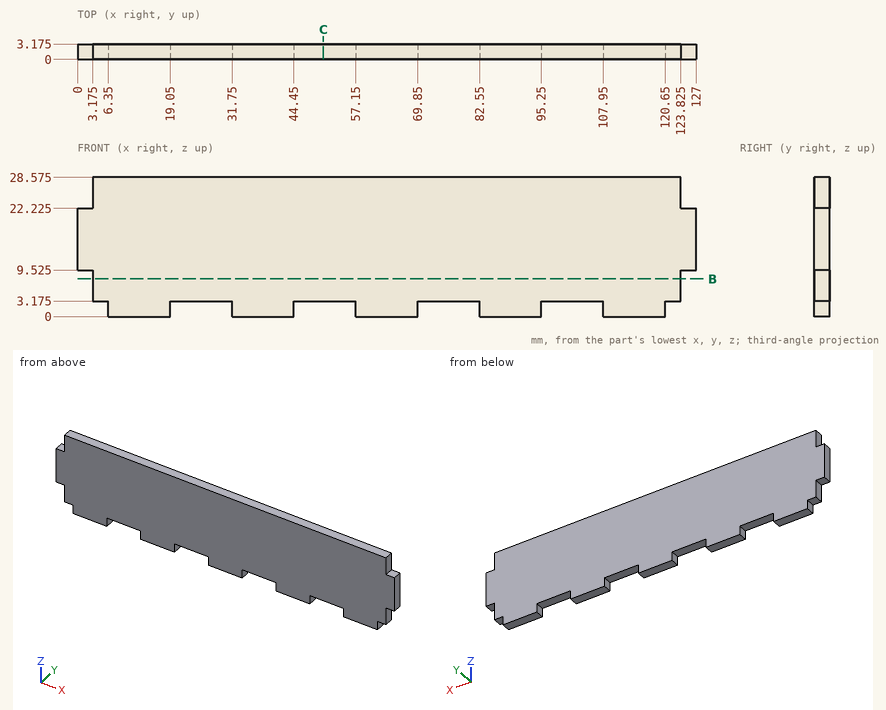
Could you check a few things on this drawing? It's one solid part, dimensions in mm from its lowest x, y, z. Give positions to 0.01 mm unless a question says otherwise; leave off trailing zeros. Loops run counter-clockwise (first coordinate to the right, second up) from the corner with the lowest first, then second, coordinate; pieces in that order, holes last. Notation, with made-up numbers: M -8.75,21 L -4.75,21 A23 cw -4.75,43 Z; hole C 10,-12 d9. An arc over 180 degrees is marked long. Answer as a JSON object with one key per item and string values.
Q1. Suppose I cut it at C-C, the plane x = 50.5. List the corners of the cut face in (y, z) for me (3 decimals).
Values found:
{"outline": "M 0,3.175 L 3.175,3.175 L 3.175,28.575 L 0,28.575 Z"}
Q2. Suppose I cut it at B-B, the plane z = 7.75. List the corners of the cut face in (x, y) for me (3 decimals).
Values found:
{"outline": "M 3.175,0 L 123.825,0 L 123.825,3.175 L 3.175,3.175 Z"}
Q3. For P1, Ø1, axis at x = 78, y = 0.5, coming from the -Z side (3 decimals); P2, Ø1.5, axis at y = 1.5, z = 3.5, coming from the -X side (3 decimals); P3, Ø1, axis at x = 2, y = 1.5, coming from the -Z side (3 decimals), each with a flat end and sliding along its axis, tell me the tip position at first contact or that it passes through.
Values found:
{"P1": "stops at z = 3.175", "P2": "stops at x = 3.175", "P3": "stops at z = 9.525"}
Q4. If I drill on probe 1 along X at (y, z) = (1.1, 3); probe 2 along Z at (x, y) = (28, 2.5) (3 decimals); probe 3 along X at (y, z) = (2, 8.75) (3 decimals), over which ranges is the centre line in solid material (lowest first)? Write a range as [from, to].
Values found:
{"probe 1": "x = [6.35, 19.05], [31.75, 44.45], [57.15, 69.85], [82.55, 95.25], [107.95, 120.65]", "probe 2": "z = [3.175, 28.575]", "probe 3": "x = [3.175, 123.825]"}
